Source: CAD feature listing. Evaluate the final solid. Frame: model axes, mm. Face numbers are marked on the shaded views. A direction names the side the tool comes from. Give positions to 0.01 mm unless a question says otherwise; leave off trailing zeros. Order: outer loops, then holes, each group sorted by start corner. A loop starts at its lowest first (then second) coordinate and runs counter-clockwise, first axis right, second up.
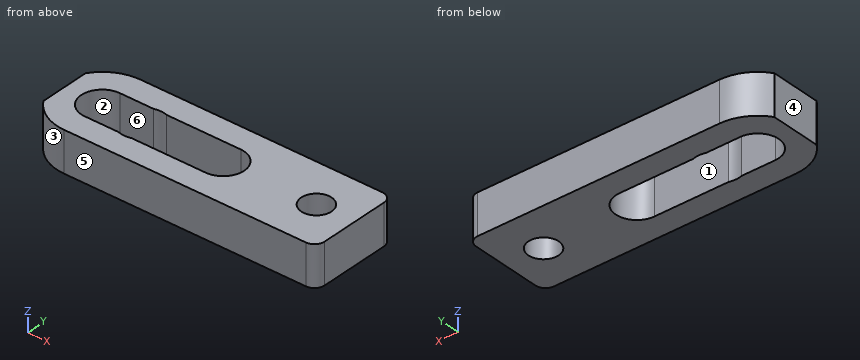
from build123d import *

# Parameters (mm, degrees)
SKETCH_R          = 3
PAD_DEPTH         = 4
SKETCH001_R       = 4.35
POCKET_DEPTH      = 4.001
POCKET_DEPTH_BACK = -4.001


with BuildPart() as part:
    # Sketch → Pad (new body, symmetric)
    with BuildSketch(Plane.XY):
        with BuildLine():
            Line((-24, 9), (24, 9))
            ThreePointArc((26, 7), (25.414214, 8.414214), (24, 9))
            Line((26, 7), (26, -7))
            ThreePointArc((24, -9), (25.414214, -8.414214), (26, -7))
            Line((24, -9), (-24, -9))
            ThreePointArc((-31.499988, -4.974955), (-28.255902, -7.930151), (-24, -9))
            Line((-31.499988, 4.974955), (-31.499988, -4.974955))
            ThreePointArc((-24, 9), (-28.255902, 7.930151), (-31.499988, 4.974955))
        make_face()
        with Locations((18.5, 0)):
            Circle(SKETCH_R, mode=Mode.SUBTRACT)
        with BuildLine():
            ThreePointArc((1.2e-05, -4.15), (4.15, 6e-06), (0, 4.15))
            Line((0, 4.15), (-24, 4.15))
            ThreePointArc((-24, 4.15), (-28.15, 0), (-24, -4.15))
            Line((-24, -4.15), (1.2e-05, -4.15))
        make_face(mode=Mode.SUBTRACT)
    extrude(amount=PAD_DEPTH, both=True)

    # Sketch001 → Pocket (cut, two sides)
    with BuildSketch(Plane.XY) as pocket_sk:
        with Locations((-16, 0)):
            Circle(SKETCH001_R)
    extrude(amount=-POCKET_DEPTH, mode=Mode.SUBTRACT)
    extrude(pocket_sk.sketch, amount=-POCKET_DEPTH_BACK, mode=Mode.SUBTRACT)


solid = part.part
1) Reachability of the marked faces 5 and 6 from +Z, -Z, +X, -X, +Y, -Y: full face, straight path, thin tool, end or side. Return the list, or none.
Checks:
face 5: +Z, -Z, +X, -X, -Y
face 6: +Z, -Z
2) Pull-direction query (Y, two-part tool) for the marked faces 1, 2, 3 and 4; classes: +Y half, -Y half, draft (parallel to the pull), parting line (faces both ways), or undercut.
Checks:
face 1: undercut
face 2: undercut
face 3: -Y half
face 4: draft
3) First-contact query: pin 1 Ø2 at (x, y) = (19.5, 1.5) entering from +Z (1 decimal). Flat tip, straight axial feed; report the tip coordinate or a pass-through.
Checks:
pin 1: passes through
4) Section query D-D on x = 18.5. Output: boundary loops of the cut face in (y, z).
Checks:
outline: (-9, -4) - (-3, -4) - (-3, 4) - (-9, 4) - close; (3, -4) - (9, -4) - (9, 4) - (3, 4) - close
5) Section query A-A on y = 0. Output: boundary loops of the cut face in (x, z), and give its area (3 significant figures).
Checks:
outline: (-31.5, -4) - (-28.15, -4) - (-28.15, 4) - (-31.5, 4) - close; (4.15, -4) - (15.5, -4) - (15.5, 4) - (4.15, 4) - close; (21.5, -4) - (26, -4) - (26, 4) - (21.5, 4) - close
area: 154 mm2
6) Ray query, L1, parallel to Y at x = -2, z = -1.75; L2, parallel to Y at x = 18.5, z = 1; L3, parallel to X at y = 2.5, z = -0.25. Return the intervals inside material, ascending.
Checks:
L1: y = -9 to -4.15, 4.15 to 9
L2: y = -9 to -3, 3 to 9
L3: x = -31.5 to -27.31, 3.31 to 16.84, 20.16 to 26
7) Section query C-C on z = -2.5. Output: boundary loops of the cut face in (x, y).
Checks:
outline: (-31.5, -4.97) arc R9 ccw to (-24, -9) - (24, -9) arc R2 ccw to (26, -7) - (26, 7) arc R2 ccw to (24, 9) - (-24, 9) arc R9 ccw to (-31.5, 4.97) - close; hole (-24, -4.15) - (-17.3, -4.15) arc R4.35 ccw to (-14.7, -4.15) - (0, -4.15) arc R4.15 ccw to (0, 4.15) - (-14.7, 4.15) arc R4.35 ccw to (-17.3, 4.15) - (-24, 4.15) arc R4.15 ccw to start; hole circle Ø6 at (18.5, 0)
8) Section query B-B on x = -14. Output: boundary loops of the cut face in (y, z).
Checks:
outline: (-9, -4) - (-4.15, -4) - (-4.15, 4) - (-9, 4) - close; (4.15, -4) - (9, -4) - (9, 4) - (4.15, 4) - close
